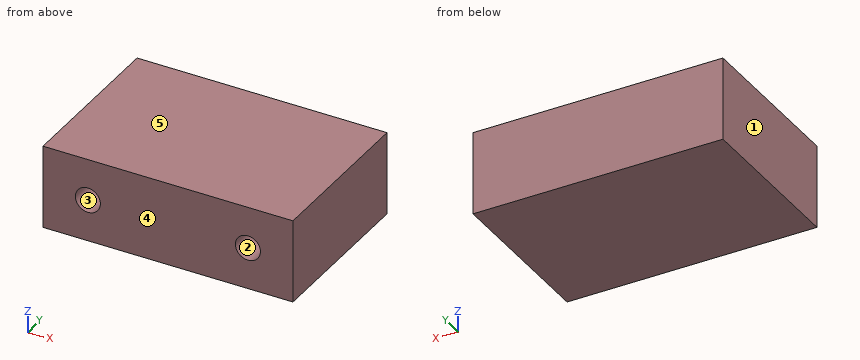
```python
from build123d import *

# Parameters (mm, degrees)
F0_W     = 30
F0_H     = 10
F1_DEPTH = 20
F3_R     = 1.5
F4_DEPTH = 10
F5_DEPTH = 10


with BuildPart() as f1:
    # F0 (on Front) → F1 (new body)
    with BuildSketch(Plane.XZ):
        Rectangle(F0_W, F0_H)
    extrude(amount=F1_DEPTH)

    # F3 (on face) → F4 (cut)
    with BuildSketch(Plane.XZ.offset(20)):
        with Locations((9.597428, 0)):
            Circle(F3_R)
    extrude(amount=-F4_DEPTH, mode=Mode.SUBTRACT)

    # F3 (on face) → F5 (cut)
    with BuildSketch(Plane.XZ.offset(20)):
        with Locations((-9.612025, 0)):
            Circle(F3_R)
    extrude(amount=-F5_DEPTH, mode=Mode.SUBTRACT)


solid = f1.part
```
The listing builds one solid part. Answer for the finished solid, in the listing's coordinates (mm). Face numbers are marked on the shaded views. A direction names the side the tool comes from. Give positions to 0.01 mm unless a question says otherwise; leave off trailing zeros. Write each loop counter-clockwise with the first axis right and the second up, starting at its lowest first coordinate (ties: lowest second). Pieces come first, ordered by that corner, then holes. Notation, with made-up numbers: (-16.75, 19.25) -> (13.25, 19.25) arc R16 ccw to (13.25, 33.25) -> close; hole circle Ø6 at (87, -26.75). An arc over 180 degrees is marked (long way). Use one line per item in the form item = value.
1) Section A-A on z = 0 is taken. Write down the section's boundary in (x, y), plus the area to 3 significant figures.
Result:
outline = (-15, -20) -> (-11.11, -20) -> (-11.11, -10) -> (-8.11, -10) -> (-8.11, -20) -> (8.1, -20) -> (8.1, -10) -> (11.1, -10) -> (11.1, -20) -> (15, -20) -> (15, 0) -> (-15, 0) -> close
area = 540 mm²
2) A tool of negligible diameter and unlimited length cuts with its end or side. For the marked faces 1 and 2, from which of +Z, -Z, +X, -X, +Y, -Y can it reach the whole face along a straight path? Write none if from no direction.
Result:
face_1 = +Z, -Z, -X, +Y, -Y
face_2 = -Y
3) For a pull along Z with two mould halves and no side action, classify the marked faces 3, 4 and 5 as +Z half, -Z half, draft (parallel to the pull), parting line (faces both ways), or undercut.
Result:
face_3 = undercut
face_4 = draft
face_5 = +Z half
4) Section B-B on y = -14.75 is taken. Write down the section's boundary in (x, z).
Result:
outline = (-15, -5) -> (15, -5) -> (15, 5) -> (-15, 5) -> close; hole circle Ø3 at (-9.61, 0); hole circle Ø3 at (9.6, 0)
5) This flat-tipped pin is pushed along its axis until it touches: P1, Ø0.9, axis at x = 9, z = -0.5, coming from the -Y side. Where does it stop, or does it pass through?
Result:
P1 = -10
6) Straight lines are drawn through the part: probe 1 along X at (y, z) = (-16.5, 1); probe 2 along X at (y, z) = (-13.75, 0.25). For each, find the intervals that lie inside material, in ascending order.
Result:
probe_1 = -15 to -10.73, -8.49 to 8.48, 10.72 to 15
probe_2 = -15 to -11.09, -8.13 to 8.12, 11.08 to 15
